CAD build for the part. Positions are in the model's coordinates, mm. A direction names the side the tool comes from. Give positions to 0.01 mm unless a question says otherwise; leave off trailing zeros. Loops run counter-clockwise (first coordinate to the right, second up) from the corner with the lowest first, then second, coordinate; pieces in that order, holes last. Notation, with made-up numbers: M 23.5,44.5 L 70.5,44.5 A16 cw 70.5,73.5 Z; hole C 5.5,51.25 d5. An arc over 180 degrees is marked long. Answer as CSV lines item,"result".
```python
from build123d import *

# Parameters (mm, degrees)
F0_W     = 100
F0_H     = 75
F0_W_2   = 41
F0_H_2   = 41
F0_H_3   = 6.35
F0_W_3   = 6.35
F1_DEPTH = 6.35


with BuildPart() as f1:
    # F0 (on Top) → F1 (new body)
    with BuildSketch(Plane.XY):
        Rectangle(F0_W, F0_H)
        Rectangle(F0_W_2, F0_H_2, mode=Mode.SUBTRACT)
        with Locations((0, 40.675)):
            Rectangle(F0_W, F0_H_3)
        with Locations((-53.175, 40.675)):
            Rectangle(F0_W_3, F0_H_3)
        with Locations((0, -40.675)):
            Rectangle(F0_W, F0_H_3)
        with Locations((53.175, -40.675)):
            Rectangle(F0_W_3, F0_H_3)
        Rectangle(F0_W_2, F0_H_2)
    extrude(amount=F1_DEPTH)


solid = f1.part
```
Q1. Wall check: line 1 (X direction, y = -38, z = 5.5); line 2 (X direction, y = -18, z = 4). Give the ranges that are in metal, low to high. Write a range as [from, to].
Solution:
line 1,"x = [-50, 56.35]"
line 2,"x = [-50, 50]"
Q2. Cut at B-B (y = 3). Write the cut outline in (x, z), and give its area (3 significant figures).
Solution:
outline,"M -50,0 L 50,0 L 50,6.35 L -50,6.35 Z"
area,"635 mm²"
Q3. Mould opens along Z. For faces 4 (the flat face through (-50, -3, 3)), 5 (the flat face through (-1, 1, 6.35)), 6 (the flat face through (-1, 1, 0)) say: released by +Z, released by -Z, zero draft, split by the parting line, or undercut.
Solution:
face 4,"zero draft"
face 5,"released by +Z"
face 6,"released by -Z"
Q4. Cut at A-A (z = 1). Write the cut outline in (x, y), and give its area (3 significant figures).
Solution:
outline,"M -56.35,37.5 L -50,37.5 L -50,-43.85 L 56.35,-43.85 L 56.35,-37.5 L 50,-37.5 L 50,43.85 L -56.35,43.85 Z"
area,"8,850 mm²"
Q5. Pin check, flat tips, straight feed: P1, Ø3, axis at x = 53.5, z = 4, coming from the +Y side; P2, Ø3, axis at x = -54, z = 4, coming from the -Y side; P3, Ø3, axis at y = -8, z = 3, coming from the +X side. Stop position of each tip, or through.
Solution:
P1,"stops at y = -37.5"
P2,"stops at y = 37.5"
P3,"stops at x = 50"
Q6. Which spindle directions (+Z, -Z, +X, -X, +Y, -Y) get a long thin tool onto all of the face, cutting with end or side? Do faces 1 (the flat face through (50, 3, 3)), 2 (the flat face through (-2, 43.85, 3)), 3 (the flat face through (-53, 37.5, 3)). Say none if no direction does.
Solution:
face 1,"+Z, -Z, +X, +Y"
face 2,"+Z, -Z, +X, -X, +Y"
face 3,"+Z, -Z, -X, -Y"
